Design review of the part built by this model. Coordinates are the model's own, in mm. Coordinates: 2 decimals unless noted, no trailing zeros. Write each loop counter-clockwise with the first axis right and the second up, starting at its lowest first coordinate (ties: lowest second). Pieces come first, ordered by that corner, then holes.
Q1. For pin 1 Ø5 at (y, z) = (21, -22.5) entering from -X, flat-tipped, find the tip position at first contact; note if it passes through.
Q2. For L1, parallel to Z at x = -5, y = 26; L2, parallel to Z at x = -12.5, y = -25; L3, parallel to Y at x = 25.5, z = -14, list the stretches that pass through material, from the lowest coordinate up.
Q3. Take a section at A-A, the plane z = 20. Write out the cut boundary in (x, y), plus the area to 3 significant figures.
Q4. Take a section at B-B, the plane y = 24. Write out the cut boundary in (x, z), plus the area to 3 significant figures.
from build123d import *

# Parameters (mm, degrees)
P_IDAT_VYSUNUT_M1_DEPTH      = 30
P_IDAT_VYSUNUT_M1_DEPTH_BACK = 30
SKICA2_W                     = 60
SKICA2_H                     = 60


with BuildPart() as part:
    # Skica1 → Rotovat1 (revolve)
    with BuildSketch(Plane.XY):
        with BuildLine():
            Line((0, -40), (0, 40))
            ThreePointArc((0, 40), (40, 0), (0, -40))
        make_face()
    revolve(axis=Axis((0, -40, 0), (0, 1, 0)))


with BuildPart() as body_2:
    # Skica2 → Přidat vysunutím1 (new, two sides: drawn at the far end of the back side and taken through both)
    with BuildSketch(Plane.XY.offset(-P_IDAT_VYSUNUT_M1_DEPTH_BACK)):
        Rectangle(SKICA2_W, SKICA2_H)
    extrude(amount=P_IDAT_VYSUNUT_M1_DEPTH + P_IDAT_VYSUNUT_M1_DEPTH_BACK)


with BuildPart() as part_1:
    add(part.part)

    # Průsečík3: read off the stored shape, not the designer's step
    # Průsečík3: intersect body 2
    add(body_2.part, mode=Mode.INTERSECT)


solid = part_1.part
Responses:
1. pin 1: stops at x = -28.29
2. L1: z = -29.98 to 29.98
2. L2: z = -28.61 to 28.61
2. L3: y = -27.45 to 27.45
3. outline: (-30, -17.32) arc R34.64 ccw to (-17.32, -30) - (17.32, -30) arc R34.64 ccw to (30, -17.32) - (30, 17.32) arc R34.64 ccw to (17.32, 30) - (-17.32, 30) arc R34.64 ccw to (-30, 17.32) - close
3. area: 3,340 mm2
4. outline: (-30, -11.14) arc R32 ccw to (-11.14, -30) - (11.14, -30) arc R32 ccw to (30, -11.14) - (30, 11.14) arc R32 ccw to (11.14, 30) - (-11.14, 30) arc R32 ccw to (-30, 11.14) - close
4. area: 3,100 mm2
